The listing builds one solid part. Answer for the finished solid, in the listing's coordinates (mm). A direction names the side the tool comes from. Give positions to 0.01 mm unless a question says otherwise; leave off trailing zeros. Write each loop counter-clockwise with the first axis right and the second up, starting at its lowest first coordinate (ties: lowest second). Pieces come first, ordered by that corner, then holes.
```python
from build123d import *

# Parameters (mm, degrees)
SKETCH1_W           = 25.4
SKETCH1_H           = 25.4
BOSS_EXTRUDE1_DEPTH = 3.175
SKETCH2_W           = 15.24
SKETCH2_H           = 12.744579596
CUT_EXTRUDE1_DEPTH  = 74.44478714
SKETCH3_R           = 1.5875
BOSS_EXTRUDE4_DEPTH = 15.24


with BuildPart() as part:
    # Sketch1 → Boss-Extrude1 (new body)
    with BuildSketch(Plane(origin=(0, 0, 0), x_dir=(0, 0, -1), z_dir=(1, 0, 0))):
        with Locations((-53.44770318, -19.057479388)):
            Rectangle(SKETCH1_W, SKETCH1_H)
    extrude(amount=BOSS_EXTRUDE1_DEPTH)

    # Sketch2 → Cut-Extrude1 (cut, through all)
    with BuildSketch(Plane(origin=(3.175, 0, 0), x_dir=(0, 0, -1), z_dir=(1, 0, 0))):
        with Locations((-53.44770318, -25.38518959)):
            Rectangle(SKETCH2_W, SKETCH2_H)
    extrude(amount=-CUT_EXTRUDE1_DEPTH, mode=Mode.SUBTRACT)

    # Sketch3 → Boss-Extrude4 (add)
    with BuildSketch(Plane.XY.offset(45.82770318)):
        with Locations(Location((1.5875, -30.04486866, 0), (0, 0, 180))):
            Circle(SKETCH3_R)
    extrude(amount=BOSS_EXTRUDE4_DEPTH)


solid = part.part
```
Item 1: Which of the six approach directions +Z, -Z, +X, -X, +Y, -Y give full straight-line access (tool end or side, diameter ignored) to faces 4 (the face through (2, -31.757, 43)), 5 (the face through (2, -19.013, 54)), 6 (the face through (1.932, -28.495, 53.341))?
Conclusion:
face 4: +Z, -Z, +X, -X, -Y
face 5: +X, -X
face 6: none
Item 2: Consider probe 1 along Z at (x, y) = (2.55, -23); probe 2 along Y at (x, z) = (1.5, 56); probe 3 along Y at (x, z) = (2.5, 51.5). Determine where each line is inside the solid, lowest interval first.
Conclusion:
probe 1: z = 40.75 to 45.83, 61.07 to 66.15
probe 2: y = -31.63 to -28.46, -19.01 to -6.36
probe 3: y = -31.34 to -28.75, -19.01 to -6.36
Item 3: Determine the mould class of faces 1 (the face through (2, -23, 61.068)), 2 (the face through (0, -16, 54)), 3 (the face through (2, -31.757, 64)) for opening direction Y: pulls with the +Y half, pulls with the -Y half, needs draft (parallel to the pull), parting line crosses it, or undercut.
Conclusion:
face 1: undercut
face 2: needs draft
face 3: pulls with the -Y half
Item 4: This flat-tipped pin is pushed along its axis until it touches: P1, Ø1, axis at x = 1, z = 59, coming from the -Y side. Where does it stop, or does it pass through?
Conclusion:
P1: stops at y = -31.63
Item 5: A cutting plane is placed at A-A, the plane y = -20.25. Give the vertices of the cut face in (x, z) (3 decimals), plus the area to 3 significant figures.
Conclusion:
outline: (0, 40.748) - (3.175, 40.748) - (3.175, 45.828) - (0, 45.828) - close; (0, 61.068) - (3.175, 61.068) - (3.175, 66.148) - (0, 66.148) - close
area: 32.3 mm2
Item 6: A cutting plane is placed at C-C, the plane x = 1.3. Give the vertices of the cut face in (y, z).
Conclusion:
outline: (-31.76, 40.75) - (-6.36, 40.75) - (-6.36, 66.15) - (-31.76, 66.15) - (-31.76, 61.07) - (-31.61, 61.07) - (-31.61, 45.83) - (-31.76, 45.83) - close; hole (-28.48, 45.83) - (-19.01, 45.83) - (-19.01, 61.07) - (-28.48, 61.07) - close
Item 7: A cutting plane is placed at B-B, the plane z = 59.75. Give the vertices of the cut face in (x, y) (1 decimal), plus the area to 3 significant figures.
Conclusion:
outline: circle Ø3.2 at (1.6, -30); (0, -19) - (3.2, -19) - (3.2, -6.4) - (0, -6.4) - close
area: 48.1 mm2
